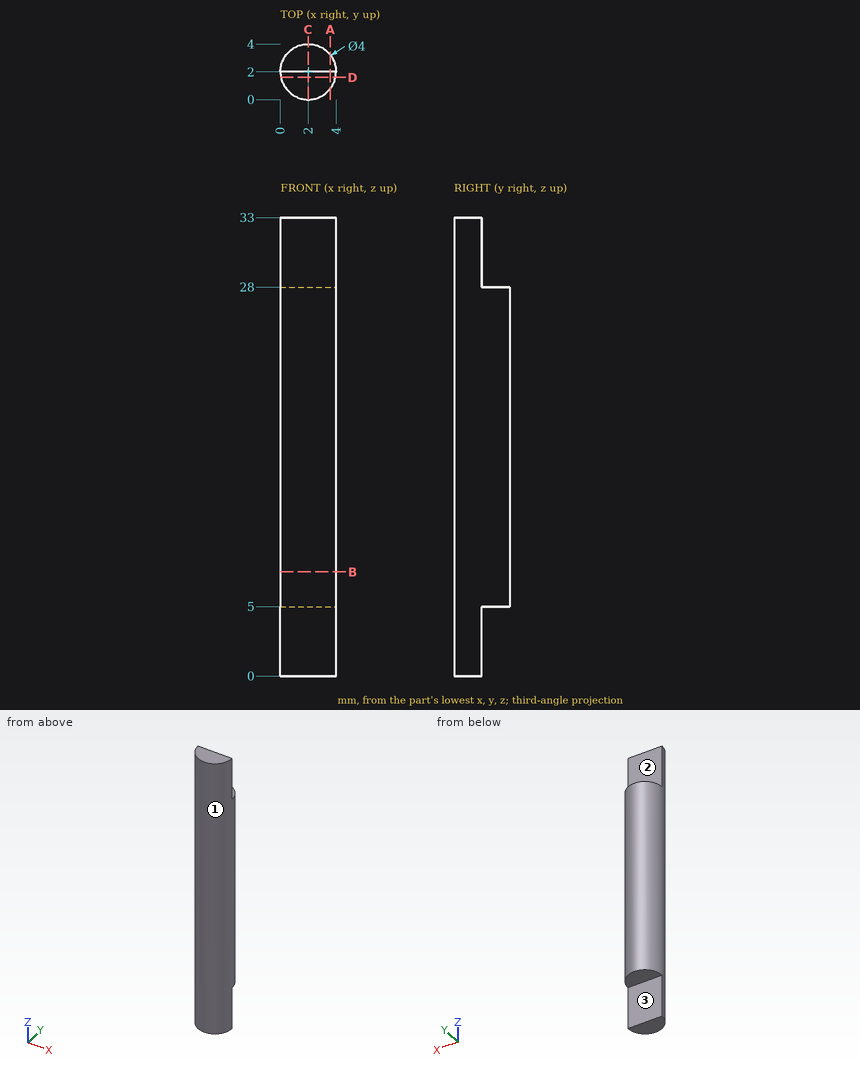
Here's the drawing with two shaded views (mm, measured from the low corner). I have some questions. A direction names the side the tool comes from. Coordinates: 2 decimals unless noted, no trailing zeros. Loops run counter-clockwise (first coordinate to the right, second up) from the corner with the lowest first, then second, coordinate; pieces in that order, holes last. Notation, with made-up numbers: (-17.5, 64) -> (5.5, 64) arc R16 ccw to (5.5, 83) -> close; hole circle Ø9 at (-4, -14). An arc over 180 degrees is marked (long way). Put each result on its own line as item: value. Start each with the question number.
Q1. For the marked faces 1, 2 and 3, which set-ups out of +Z, -Z, +X, -X, +Y, -Y let a thin tool reach every point of the face, with its end or its side?
Q2. I'm going to push flat-ended pins straight in: P1, Ø1.2, axis at x = 1.5, z = 2, coming from the +Y side; P2, Ø1, axis at y = 1, z = 23.5, coming from the -X side. Where does each tip first touch, or does it pass through?
Q3. I want a section at B-B (z = 7.5). Write out the boundary of the cut face in (x, y), plus the area to 3 significant figures.
Q4. If I drill on line 1 (Y direction, x = 1.85, z = 21); line 2 (X direction, y = 1.9, z = 31.5); line 3 (Z direction, x = 0.45, y = 2.8), over which ranges is the centre line in solid material (lowest first)? Write a range as [from, to].
Q5. I want a section at C-C (x = 2). Write out the boundary of the cut face in (y, z).
Q6. I want a section at D-D (y = 1.6). Write out the boundary of the cut face in (x, z).
Q7. I want a section at A-A (x = 3.6). Write out the boundary of the cut face in (y, z), plus the area to 3 significant figures.
Taken from the geometry:
1. face 1: +Z, -Z
1. face 2: +Z, +X, -X, +Y
1. face 3: -Z, +X, -X, +Y
2. P1: stops at y = 2
2. P2: stops at x = 0.06
3. outline: circle Ø4 at (2, 2)
3. area: 12.6 mm2
4. line 1: y = [0.01, 3.99]
4. line 2: x = [0, 4]
4. line 3: z = [5, 28]
5. outline: (0, 0) -> (2, 0) -> (2, 5) -> (4, 5) -> (4, 28) -> (2, 28) -> (2, 33) -> (0, 33) -> close
6. outline: (0.04, 0) -> (3.96, 0) -> (3.96, 33) -> (0.04, 33) -> close
7. outline: (0.8, 0) -> (2, 0) -> (2, 5) -> (3.2, 5) -> (3.2, 28) -> (2, 28) -> (2, 33) -> (0.8, 33) -> close
7. area: 67.2 mm2
